Design review of the part shown in the three views and the two pictorial views. Dimensions are in mm from the part's minimum x, y and z. A direction names the side the tool comes from. Give positions to 0.01 mm unless a question says otherwise; leave off trailing zeros. Order: outer loops, then holes, each group sorted by start corner. A loop starts at its lowest first (then second) coordinate and runs counter-clockwise, first axis right, second up.
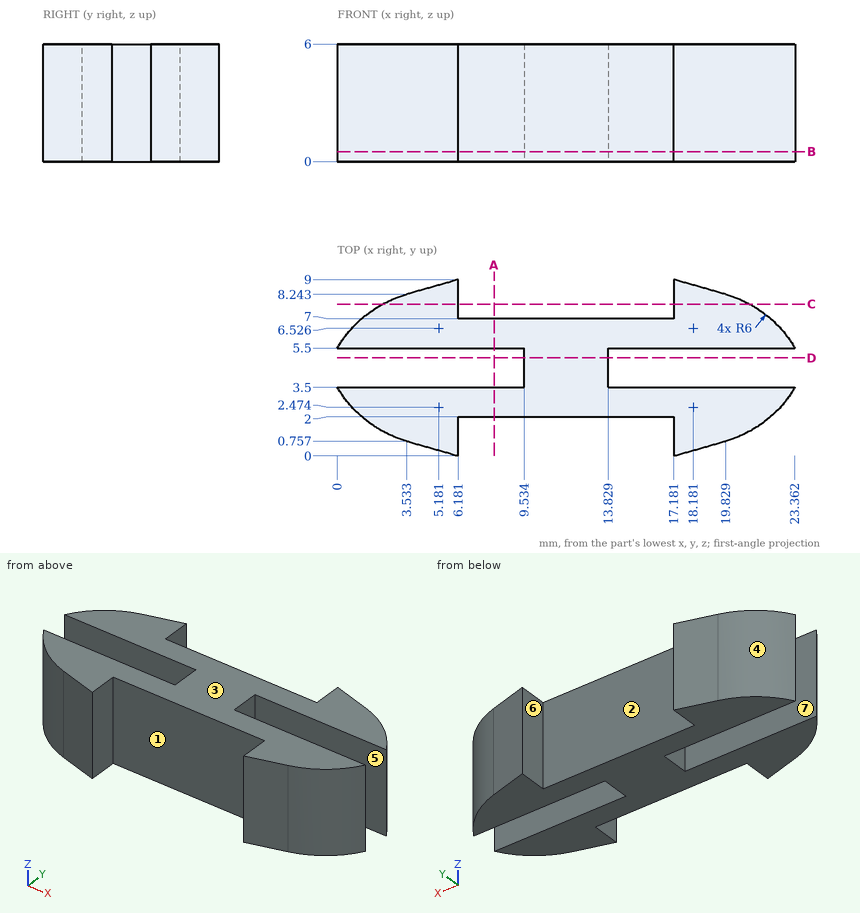
Item 1: For the marked faces 5, 6 and 7, list the 3-axis set-ups (+Z, -Z, +X, -X, +Y, -Y) from which the entire face can be reached by the end or side of a thin tool; tool diameter is ignored.
Values found:
face 5: +Z, -Z, +X
face 6: +Z, -Z, +Y
face 7: +Z, -Z, -X
Item 2: For line 1 (Y direction, x = 14.25, z = 3.5); line 2 (Y direction, x = 13.25, z = 1); line 3 (Y direction, x = 3.75, z = 1.75) (1 decimal), list the stretches that pass through material, from the lowest coordinate up.
Values found:
line 1: y = 2 to 3.5, 5.5 to 7
line 2: y = 2 to 7
line 3: y = 0.7 to 3.5, 5.5 to 8.3
Item 3: Take a section at A-A (x = 8). Give the boundary of the cut face in (y, z).
Values found:
outline: (2, 0) - (3.5, 0) - (3.5, 6) - (2, 6) - close; (5.5, 0) - (7, 0) - (7, 6) - (5.5, 6) - close
Item 4: Take a section at B-B (z = 0.5). Give the boundary of the cut face in (x, y) (1 decimal).
Values found:
outline: (0, 3.5) arc R6 ccw to (3.5, 0.8) - (6.2, 0) - (6.2, 2) - (17.2, 2) - (17.2, 0) - (19.8, 0.8) arc R6 ccw to (23.4, 3.5) - (13.8, 3.5) - (13.8, 5.5) - (23.4, 5.5) arc R6 ccw to (19.8, 8.2) - (17.2, 9) - (17.2, 7) - (6.2, 7) - (6.2, 9) - (3.5, 8.2) arc R6 ccw to (0, 5.5) - (9.5, 5.5) - (9.5, 3.5) - close
Item 5: Take a section at D-D (y = 5). Give the boundary of the cut face in (x, z).
Values found:
outline: (9.53, 0) - (13.83, 0) - (13.83, 6) - (9.53, 6) - close
Item 6: Draft analysis for pull direction X (two halves, no side actions). For the marked faces 1, 2, 3 and 4, state which applies: released by +X, released by -X, zero draft, split by the parting line, or undercut.
Values found:
face 1: undercut
face 2: undercut
face 3: zero draft
face 4: released by -X
Item 7: Clearance check with flat-ended pins moving along their axes: pin 1 Ø2 at (y, z) = (7.5, 2) entering from -X; pin 2 Ø1.5 at (x, z) = (20.5, 3.5) entering from +Y; pin 3 Ø1.6 at (y, z) = (8, 3.5) entering from +X; pin 4 Ø1.8 at (x, z) = (16.5, 3.5) entering from +Y. State where each tip first meets the part, or that it passes through.
Values found:
pin 1: stops at x = 0.73
pin 2: stops at y = 8.27
pin 3: stops at x = 21.88
pin 4: stops at y = 9
Item 8: Take a section at C-C (y = 7.75). Give the boundary of the cut face in (x, z), and give its area (3 significant figures).
Values found:
outline: (2.32, 0) - (6.18, 0) - (6.18, 6) - (2.32, 6) - close; (17.18, 0) - (21.04, 0) - (21.04, 6) - (17.18, 6) - close
area: 46.3 mm2
